Geometry: final body of the model. Coordinates: model frame, mm. A direction names the side the tool comes from. Round coordinates to 2 decimals unless told otherwise and drop trailing zeros. Loops run counter-clockwise (first coordinate to the right, second up) from the corner with the lowest first, then second, coordinate; pieces in that order, holes last. Notation, with made-up numbers: M -15.5,72.25 L 9.5,72.25 A16 cw 9.5,93.25 Z; hole C 32.25,52 d3. An arc over 180 degrees is marked long. Answer as a JSON object with one key per item and string values.
from build123d import *

# Parameters (mm, degrees)
SKETCH1_W            = 22.9
SKETCH1_H            = 20.7
BOSS_EXTRUDE1_DEPTH  = 11.63
SKETCH3_R            = 5.45
BOSS_EXTRUDE2_DEPTH  = 3.5
SKETCH4_W            = 1
SKETCH4_H            = 11.63
BOSS_EXTRUDE3_DEPTH  = 5
SKETCH5_R            = 1
CUT_EXTRUDE1_DEPTH   = 1
BOSS_EXTRUDE4_DEPTH  = 2.2
SKETCH8_R            = 0.5
BOSS_EXTRUDE6_DEPTH  = 4.5
SKETCH10_R           = 0.5
BOSS_EXTRUDE9_DEPTH  = 4.5
SKETCH9_R            = 0.5
BOSS_EXTRUDE10_DEPTH = 4.5
SKETCH13_R           = 0.5
CUT_EXTRUDE2_DEPTH   = 2.2


with BuildPart() as part:
    # Sketch1 → Boss-Extrude1 (new body)
    with BuildSketch(Plane(origin=(0, 0, 0), x_dir=(1, 0, 0), z_dir=(0, 1, 0))):
        with Locations((11.45, 10.35)):
            Rectangle(SKETCH1_W, SKETCH1_H)
    extrude(amount=BOSS_EXTRUDE1_DEPTH)

    # Sketch3 → Boss-Extrude2 (add)
    with BuildSketch(Plane(origin=(0, 0, -20.7), x_dir=(-1, 0, 0), z_dir=(0, 0, -1))):
        with Locations((-17.4, 5.815)):
            Circle(SKETCH3_R)
    extrude(amount=BOSS_EXTRUDE2_DEPTH)

    # Sketch4 → Boss-Extrude3 (add)
    with BuildSketch(Plane(origin=(22.9, 0, 0), x_dir=(0, 0, -1), z_dir=(1, 0, 0))):
        with Locations((17.7, 5.815)):
            Rectangle(SKETCH4_W, SKETCH4_H)
    boss_extrude3 = extrude(amount=BOSS_EXTRUDE3_DEPTH)

    # Sketch5 → Cut-Extrude1 (cut)
    with BuildSketch(Plane(origin=(0, 0, -18.2), x_dir=(-1, 0, 0), z_dir=(0, 0, -1))):
        with Locations((-25.9, 5.815)):
            Circle(SKETCH5_R)
    cut_extrude1 = extrude(amount=-CUT_EXTRUDE1_DEPTH, mode=Mode.SUBTRACT)

    # Mirror1: Boss-Extrude3, Cut-Extrude1 across plane
    add(boss_extrude3.mirror(Plane.ZY.offset(-11.45)))
    add(cut_extrude1.mirror(Plane.ZY.offset(-11.45)), mode=Mode.SUBTRACT)

    # Sketch6 → Boss-Extrude4 (add)
    with BuildSketch(Plane(origin=(0, 0, -24.2), x_dir=(-1, 0, 0), z_dir=(0, 0, -1))):
        Polygon((-17.4, 7.815), (-17.728528158, 7.466622583), (-18.165366865, 7.662759065), (-18.33556904, 7.215178017), (-18.814213562, 7.229213562), (-18.800178017, 6.75056904), (-19.247759065, 6.580366865), (-19.051622583, 6.143528158), (-19.4, 5.815), (-19.051622583, 5.486471842), (-19.247759065, 5.049633135), (-18.800178017, 4.87943096), (-18.814213562, 4.400786438), (-18.33556904, 4.414821983), (-18.165366865, 3.967240935), (-17.728528158, 4.163377417), (-17.4, 3.815), (-17.071471842, 4.163377417), (-16.634633135, 3.967240935), (-16.46443096, 4.414821983), (-15.985786438, 4.400786438), (-15.999821983, 4.87943096), (-15.552240935, 5.049633135), (-15.748377417, 5.486471842), (-15.4, 5.815), (-15.748377417, 6.143528158), (-15.552240935, 6.580366865), (-15.999821983, 6.75056904), (-15.985786438, 7.229213562), (-16.46443096, 7.215178017), (-16.634633135, 7.662759065), (-17.071471842, 7.466622583), align=None)
    extrude(amount=BOSS_EXTRUDE4_DEPTH)

    # Sketch8 → Boss-Extrude6 (add)
    with BuildSketch(Plane(origin=(22.9, 0, 0), x_dir=(0, 0, -1), z_dir=(1, 0, 0))):
        with Locations((4, 5.815)):
            Circle(SKETCH8_R)
    extrude(amount=BOSS_EXTRUDE6_DEPTH)

    # Sketch10 → Boss-Extrude9 (add)
    with BuildSketch(Plane(origin=(22.9, 0, 0), x_dir=(0, 0, -1), z_dir=(1, 0, 0))):
        with Locations((4, 4.805)):
            Circle(SKETCH10_R)
    extrude(amount=BOSS_EXTRUDE9_DEPTH)

    # Sketch9 → Boss-Extrude10 (add)
    with BuildSketch(Plane(origin=(22.9, 0, 0), x_dir=(0, 0, -1), z_dir=(1, 0, 0))):
        with Locations((4, 6.825)):
            Circle(SKETCH9_R)
    extrude(amount=BOSS_EXTRUDE10_DEPTH)

    # Sketch13 → Cut-Extrude2 (cut)
    with BuildSketch(Plane(origin=(0, 0, -26.4), x_dir=(-1, 0, 0), z_dir=(0, 0, -1))):
        with Locations((-17.4, 5.815)):
            Circle(SKETCH13_R)
    extrude(amount=-CUT_EXTRUDE2_DEPTH, mode=Mode.SUBTRACT)


solid = part.part
1) Section query B-B (z = -4). Return the cut outline in (x, y) (3 decimals), and give its area (3 significant figures).
Results:
{"outline": "M 0,0 L 22.9,0 L 22.9,4.305 L 27.4,4.305 L 27.4,5.305 L 22.9,5.305 L 22.9,5.315 L 27.4,5.315 L 27.4,6.315 L 22.9,6.315 L 22.9,6.325 L 27.4,6.325 L 27.4,7.325 L 22.9,7.325 L 22.9,11.63 L 0,11.63 Z", "area": "280 mm2"}
2) Ray query, line 1 (Y direction, x = 26, z = -17.25); line 2 (X direction, y = 4, z = -8.25); line 3 (X direction, y = 6.5, z = -17.5). Return the intervals inside material, ascending.
Results:
{"line 1": "0 to 4.82, 6.81 to 11.63", "line 2": "0 to 22.9", "line 3": "-5 to -3.73, -2.27 to 25.17, 26.63 to 27.9"}
3) Section query D-D (y = 10.75). Return the cut outline in (x, z).
Results:
{"outline": "M -5,-18.2 L 0,-18.2 L 0,-20.7 L 15.09,-20.7 L 15.09,-24.2 L 19.71,-24.2 L 19.71,-20.7 L 22.9,-20.7 L 22.9,-18.2 L 27.9,-18.2 L 27.9,-17.2 L 22.9,-17.2 L 22.9,0 L 0,0 L 0,-17.2 L -5,-17.2 Z"}
4) Section query C-C (x = -3). Return the cut outline in (y, z) (3 decimals), and give its area (3 significant figures).
Results:
{"outline": "M 0,-18.2 L 4.815,-18.2 L 4.815,-17.2 L 0,-17.2 Z; M 6.815,-18.2 L 11.63,-18.2 L 11.63,-17.2 L 6.815,-17.2 Z", "area": "9.63 mm2"}
5) Pin query (flat end, axial travel): P1, Ø4, axis at y = 1, z = -5.5, coming from the -X side; P2, Ø0.5, axis at x = 17.5, y = 6, coming from the -Z side; P3, Ø1.2, axis at x = 25.9, y = 5.815, coming from the +Z side. Return the tip coordinate at first contact, or that it passes through.
Results:
{"P1": "x = 0", "P2": "z = -24.2", "P3": "z = -3.5"}
6) Pull-direction query (Z, two-part tool) for faces 4 (the cylindrical face through (25.12, 7.32, -3.93)), 5 (the flat face through (27.4, 5, -4)), 6 (the flat face through (9, 6, -20.7)); classes: +Z half, -Z half, draft (parallel to the pull), parting line (faces both ways), or undercut.
Results:
{"face 4": "undercut", "face 5": "draft", "face 6": "-Z half"}
7) Section query A-A (x = 25.9). Return the cut outline in (y, z) (3 decimals), and give its area (3 significant figures).
Results:
{"outline": "M 0,-18.2 L 4.815,-18.2 L 4.815,-17.2 L 0,-17.2 Z; C 4.805,-4 d1; C 5.815,-4 d1; C 6.825,-4 d1; M 6.815,-18.2 L 11.63,-18.2 L 11.63,-17.2 L 6.815,-17.2 Z", "area": "12.0 mm2"}
8) Reachability of faces 1 (the flat face through (17.4, 5.8, -24.2)), 2 (the flat face through (27.4, 6, -4)), 3 (the flat face through (22.9, 6, -19)) from +Z, -Z, +X, -X, +Y, -Y: full face, straight path, thin tool, end or side. Return the list, or none.
Results:
{"face 1": "-Z", "face 2": "+Z, +X, +Y, -Y", "face 3": "-Z, +X, +Y, -Y"}
